```python
from build123d import *

# Parameters (mm, degrees)
SKETCH1_R           = 2.475
SKETCH1_R_2         = 4.025
SKETCH1_R_3         = 21
BOSS_EXTRUDE1_DEPTH = 10
SKETCH1_5_R         = 4.25
BOSS_EXTRUDE4_DEPTH = 10
SKETCH1_4_R         = 21
SKETCH1_4_R_2       = 13.5
BOSS_EXTRUDE2_DEPTH = 5
FILLET1_R           = 10


with BuildPart() as part:
    # Sketch1 → Boss-Extrude1 (new body)
    with BuildSketch(Plane(origin=(0, 0, 0), x_dir=(1, 0, 0), z_dir=(0, 1, 0))):
        with BuildLine():
            ThreePointArc((0, 65), (-65, 0), (0, -65))
            Line((0, -65), (150, -65))
            Line((150, -65), (150, 65))
            Line((150, 65), (0, 65))
        make_face()
        with BuildLine():
            ThreePointArc((45.5, -42), (48, -39.5), (50.5, -42))
            Line((50.5, -42), (50.5, -52))
            ThreePointArc((50.5, -52), (48, -54.5), (45.5, -52))
            Line((45.5, -52), (45.5, -42))
        make_face(mode=Mode.SUBTRACT)
        with Locations(Location((0, -60, 0), (0, 0, 270))):
            Circle(SKETCH1_R, mode=Mode.SUBTRACT)
        with Locations(Location((-60, 0, 0), (0, 0, 270))):
            Circle(SKETCH1_R, mode=Mode.SUBTRACT)
        with Locations(Location((0, 60, 0), (0, 0, 270))):
            Circle(SKETCH1_R, mode=Mode.SUBTRACT)
        with Locations(Location((60, 0, 0), (0, 0, 270))):
            Circle(SKETCH1_R, mode=Mode.SUBTRACT)
        with Locations(Location((140, 0, 0), (0, 0, 270))):
            Circle(SKETCH1_R_2, mode=Mode.SUBTRACT)
        with BuildLine():
            ThreePointArc((45.5, 6), (48, 8.5), (50.5, 6))
            Line((50.5, 6), (50.5, -4))
            ThreePointArc((50.5, -4), (48, -6.5), (45.5, -4))
            Line((45.5, -4), (45.5, 6))
        make_face(mode=Mode.SUBTRACT)
        with BuildLine():
            ThreePointArc((-40.5, -24.604436172), (-40.518742246, -24.42765838), (-40.525, -24.25))
            Line((-40.525, -24.25), (-40.525, -21.75))
            ThreePointArc((-40.525, -21.75), (-40.518742246, -21.57234162), (-40.5, -21.395563828))
            Line((-40.5, -21.395563828), (-40.5, -18))
            ThreePointArc((-40.5, -18), (-38, -15.5), (-35.5, -18))
            Line((-35.5, -18), (-35.5, -21.395563828))
            ThreePointArc((-35.5, -21.395563828), (-35.481257754, -21.57234162), (-35.475, -21.75))
            Line((-35.475, -21.75), (-35.475, -24.25))
            ThreePointArc((-35.475, -24.25), (-35.481257754, -24.42765838), (-35.5, -24.604436172))
            Line((-35.5, -24.604436172), (-35.5, -28))
            ThreePointArc((-35.5, -28), (-38, -30.5), (-40.5, -28))
            Line((-40.5, -28), (-40.5, -24.604436172))
        make_face(mode=Mode.SUBTRACT)
        with Locations(Location((0, 0, 0), (0, 0, 270))):
            Circle(SKETCH1_R_3, mode=Mode.SUBTRACT)
    extrude(amount=BOSS_EXTRUDE1_DEPTH)

    # Sketch1_5 → Boss-Extrude4 (add)
    with BuildSketch(Plane(origin=(0, 0, 0), x_dir=(1, 0, 0), z_dir=(0, 1, 0))):
        with BuildLine():
            ThreePointArc((0, 65), (-65, 0), (0, -65))
            Line((0, -65), (-85, -65))
            Line((-85, -65), (-85, 65))
            Line((-85, 65), (0, 65))
        make_face()
        with Locations(Location((-77, 0, 0), (0, 0, 270))):
            Circle(SKETCH1_5_R, mode=Mode.SUBTRACT)
    extrude(amount=BOSS_EXTRUDE4_DEPTH)

    # Sketch1_4 → Boss-Extrude2 (add)
    with BuildSketch(Plane(origin=(0, 0, 0), x_dir=(1, 0, 0), z_dir=(0, 1, 0))):
        with Locations(Location((0, 0, 0), (0, 0, 270))):
            Circle(SKETCH1_4_R)
        with Locations(Location((0, 0, 0), (0, 0, 270))):
            Circle(SKETCH1_4_R_2, mode=Mode.SUBTRACT)
    extrude(amount=BOSS_EXTRUDE2_DEPTH)

    # Fillet1
    fillet1_edges = [part.edges().sort_by_distance(p)[0] for p in [
        (150, 5, -65),
        (150, 5, 65),
        (-85, 5, -65),
        (-85, 5, 65),
    ]]
    fillet(fillet1_edges, radius=FILLET1_R)


solid = part.part
```
Work out the finished part from the listing and answer in its coordinate system (mm). A direction names the side the tool comes from. Round coordinates to 2 decimals unless told otherwise and drop trailing zeros. Write each loop counter-clockwise with the first axis right and the second up, starting at its lowest first coordinate (ties: lowest second). Pieces come first, ordered by that corner, then holes.
1) Determine the mould class of faces 1 (the face through (34, 0, -1)), 2 (the face through (45.5, 5, -1)), 3 (the face through (146.99, 5.07, -62.15)), 4 (the face through (-38.1, 4.9, 15.5)) for opening direction Z: pulls with the +Z half, pulls with the -Z half, needs draft (parallel to the pull), parting line crosses it, or undercut.
2) A cutting plane is placed at A-A on x = -38. Determine the outline of the cut face in (y, z), and give its area (3 significant figures).
3) A cutting plane is placed at B-B on z = 0. Give the number of separate pieces and of enclosed holes in the cut face, and give its area (3 significant figures).
4) Consider probe 1 along X at (y, z) = (3.5, 24.5); probe 2 along X at (y, z) = (4, 60) (3 decimals); probe 3 along Z at (x, y) = (58.5, 7.5). Determine where each line is inside the solid, lowest interval first.
5) Which of the six approach directions +Z, -Z, +X, -X, +Y, -Y give full straight-line access (tool end or side, diameter ignored) to faces 5 (the face through (50.5, 5, -1)), 6 (the face through (6.31, 7.46, 20.03)), 7 (the face through (34, 5, 65))?
6) A cutting plane is placed at C-C on x = 0. Determine the outline of the cut face in (y, z) (3 decimals), and give its area (3 significant figures).
Entries:
1. face 1: needs draft
1. face 2: undercut
1. face 3: pulls with the -Z half
1. face 4: undercut
2. outline: (0, -65) - (10, -65) - (10, 15.5) - (0, 15.5) - close; (0, 30.5) - (10, 30.5) - (10, 65) - (0, 65) - close
2. area: 1,150 mm2
3. separate pieces: 7
3. enclosed holes: 0
3. area: 1,690 mm2
4. probe 1: x = -85 to -40.51, -35.49 to 150
4. probe 2: x = -83.66 to -2.475, 2.475 to 148.66
4. probe 3: z = -65 to -1.97, 1.97 to 65
5. face 5: +Y, -Y
5. face 6: +Y
5. face 7: +Z, +X, -X, +Y, -Y
6. outline: (0, -65) - (10, -65) - (10, -62.475) - (0, -62.475) - close; (0, -57.525) - (10, -57.525) - (10, -21) - (5, -21) - (5, -13.5) - (0, -13.5) - close; (0, 13.5) - (5, 13.5) - (5, 21) - (10, 21) - (10, 57.525) - (0, 57.525) - close; (0, 62.475) - (10, 62.475) - (10, 65) - (0, 65) - close
6. area: 856 mm2
